from build123d import *

# Parameters (mm, degrees)
F0_R     = 63.5
F2_W     = 127
F2_H     = 127
F4_R     = 31.75
F5_DEPTH = 25.4
F7_DEPTH = 127


with BuildPart() as f3:
    # F0 (on Front) → F3 section 0
    with BuildSketch(Plane.XZ):
        Circle(F0_R)
    # F2 (on offset) → F3 section 1
    with BuildSketch(Plane.XZ.offset(101.6)):
        Rectangle(F2_W, F2_H)
    loft()

    # F4 (on face) → F5 (join)
    with BuildSketch(Plane.XZ.offset(101.6)):
        Circle(F4_R)
    extrude(amount=F5_DEPTH)

    # F6 (on face) → F7 (cut)
    with BuildSketch(Plane.XZ.offset(127)):
        Polygon((-22.394618, 7.276453), (-13.840635, -19.05), (13.840635, -19.05), (22.394618, 7.276453), (0, 23.547095), align=None)
    extrude(amount=-F7_DEPTH, mode=Mode.SUBTRACT)


solid = f3.part
Could you check a few things on this model? Use its own coordinates, in mm. A direction names the side the tool comes from. Give positions to 0.01 mm unless a question says otherwise; leave off trailing zeros. Write each loop counter-clockwise with the first axis right and the second up, starting at its lowest first coordinate (ties: lowest second). Pieces come first, ordered by that corner, then holes. Notation, with made-up numbers: (28.25, 56) -> (34.25, 56) arc R17 cw to (34.25, 74) -> close; hole circle Ø6 at (5, 53). An arc over 180 degrees is marked (long way). Answer as CSV lines item,"result". Start each with the question number.
(1) Please list where these lines run through material, in increasing order: line 1 (Y direction, x = -29, z = 31.5); line 2 (X direction, y = -20, z = -6); line 3 (Z direction, x = -8, y = -37).
(2) Which directions (+Z, -Z, +X, -X, +Y, -Y) give clear straight access to the entire face, cutting with the end or side of a thin tool? Please do faces 4 (the face through (0, -127, -21)), 5 (the face through (-11.041, -64.389, 15.526)), 6 (the face through (-16, -101.6, -35)).
(3) If we section it at A-A, the plane y = -119: Write out the boundary of the cut face in (x, z), and give its area (3 significant figures).
(4) If we mould it in two halves opening along Z, with no side actions, what happens to faces 1 (the face through (-6.883, -114.122, -30.995)), 2 (the face through (11.35, -64.39, 15.3)), 3 (the face through (13, 0, 15))? For each: +Z half, -Z half, draft (parallel to the pull), parting line (faces both ways), or undercut.
(5) I'm going to push flat-ended pins straight in: pin 1 Ø10 at (y, z) = (-22.5, -36) entering from +X; pin 2 Ø1 at (y, z) = (-64, 42) entering from +X; pin 3 Ø1.5 at (y, z) = (-70.5, 49) entering from +X. Where does each tip first touch, or does it pass through?
Answer list:
1,line 1,"-101.6 to 0"
1,line 2,"-63.29 to -18.08, 18.08 to 63.29"
1,line 3,"-63.23 to -19.05, 17.73 to 63.23"
2,face 4,"+Z, -Z, +X, -X, -Y"
2,face 5,"+Y, -Y"
2,face 6,"-Y"
3,outline,"circle Ø63.5 at (0, 0); hole (-22.39, 7.28) -> (-13.84, -19.05) -> (13.84, -19.05) -> (22.39, 7.28) -> (0, 23.55) -> close"
3,area,"1,850 mm^2"
4,face 1,"parting line"
4,face 2,"undercut"
4,face 3,"draft"
5,pin 1,"x = 58.14"
5,pin 2,"x = 59.84"
5,pin 3,"x = 59.58"
